Geometry: see drawing. Coordinates: mm, zero at the bounding-box minimum. Give positions to 0.01 mm unless a question says otherwise; leave off trailing zeros. Write each loop counter-clockwise with the first axis right and the second up, starting at its lowest first coordinate (ties: lowest second). Pieces come first, ordered by that corner, then holes. Notation, with made-up numbers: (-25.75, -37) - (-12.75, -37) arc R19 ccw to (-12.75, -14) - close; hole circle Ø8 at (30.25, -10). An arc over 180 degrees is marked (long way). One line per question, with ' | ' between items. Start each with the question number.
(1) Section D-D, the plane x = 2.5. Return loops of the section in (y, z), plus the area to 3 significant figures.
(2) Ray query, line 1 (Z direction, x = 15, y = 7.8); line 2 (Z direction, x = 22, y = 6.5); line 3 (Y direction, x = 27, z = 29). Return the intervals inside material, ascending. Write a range as [from, to].
(3) Section B-B, the plane z = 22. Return loops of the section in (x, y), plus the area to 3 significant figures.
(4) Section A-A, the plane y = 6.5. Return loops of the section in (x, z), plus the area to 3 significant figures.
(5) Section C-C, the plane x = 15. Return loops of the section in (y, z).
(6) Pin query (flat end, axial travel): pin 1 (3.5 mm diameter, centred on x = 15, z = 22, fed in from -Y). Return the tip coordinate at first contact, or that it passes through.
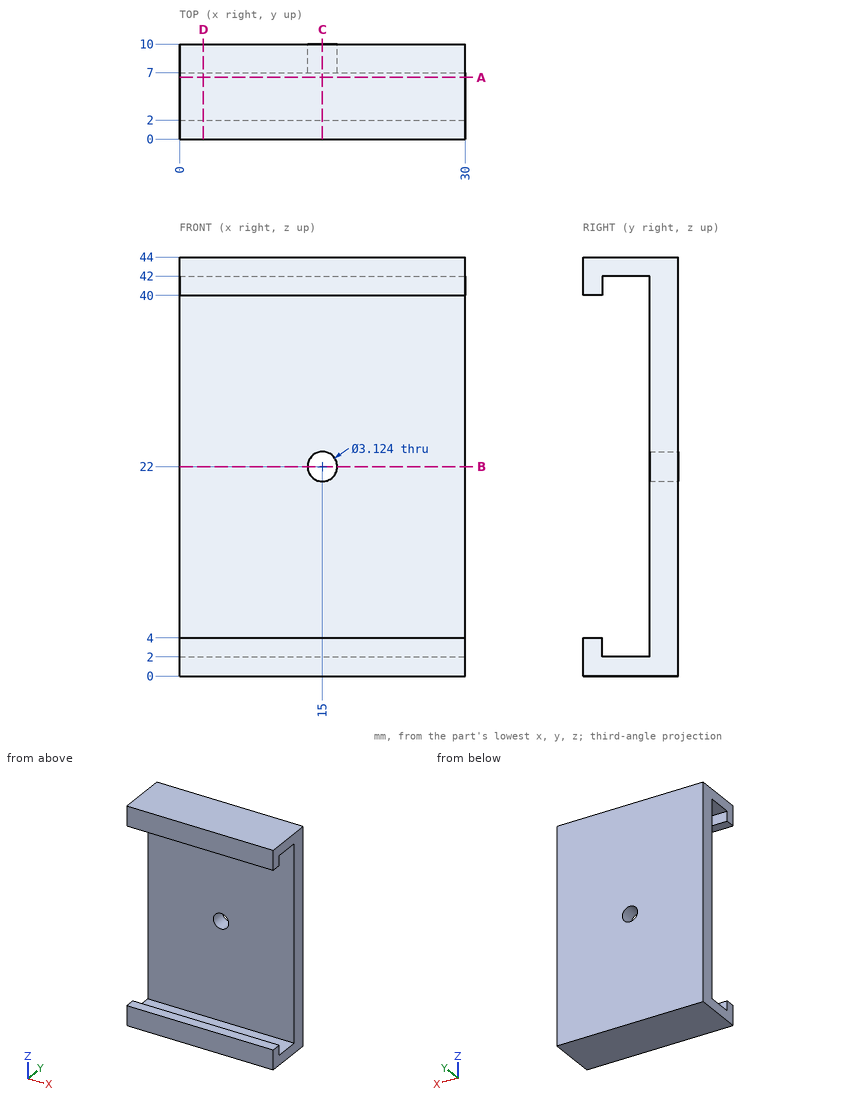
Check sheet entries:
1) outline: (0, 0) - (10, 0) - (10, 44) - (0, 44) - (0, 40) - (2, 40) - (2, 42) - (7, 42) - (7, 2) - (2, 2) - (2, 4) - (0, 4) - close | area: 168 mm²
2) line 1: [0, 20.44], [23.56, 44] | line 2: [0, 2], [42, 44] | line 3: [7, 10]
3) outline: (0, 7) - (13.44, 7) - (13.44, 10) - (0, 10) - close; (16.56, 7) - (30, 7) - (30, 10) - (16.56, 10) - close | area: 80.6 mm²
4) outline: (0, 0) - (30, 0) - (30, 2) - (0, 2) - close; (0, 42) - (30, 42) - (30, 44) - (0, 44) - close | area: 120 mm²
5) outline: (0, 0) - (10, 0) - (10, 20.44) - (7, 20.44) - (7, 2) - (2, 2) - (2, 4) - (0, 4) - close; (0, 40) - (2, 40) - (2, 42) - (7, 42) - (7, 23.56) - (10, 23.56) - (10, 44) - (0, 44) - close
6) pin 1: y = 7
